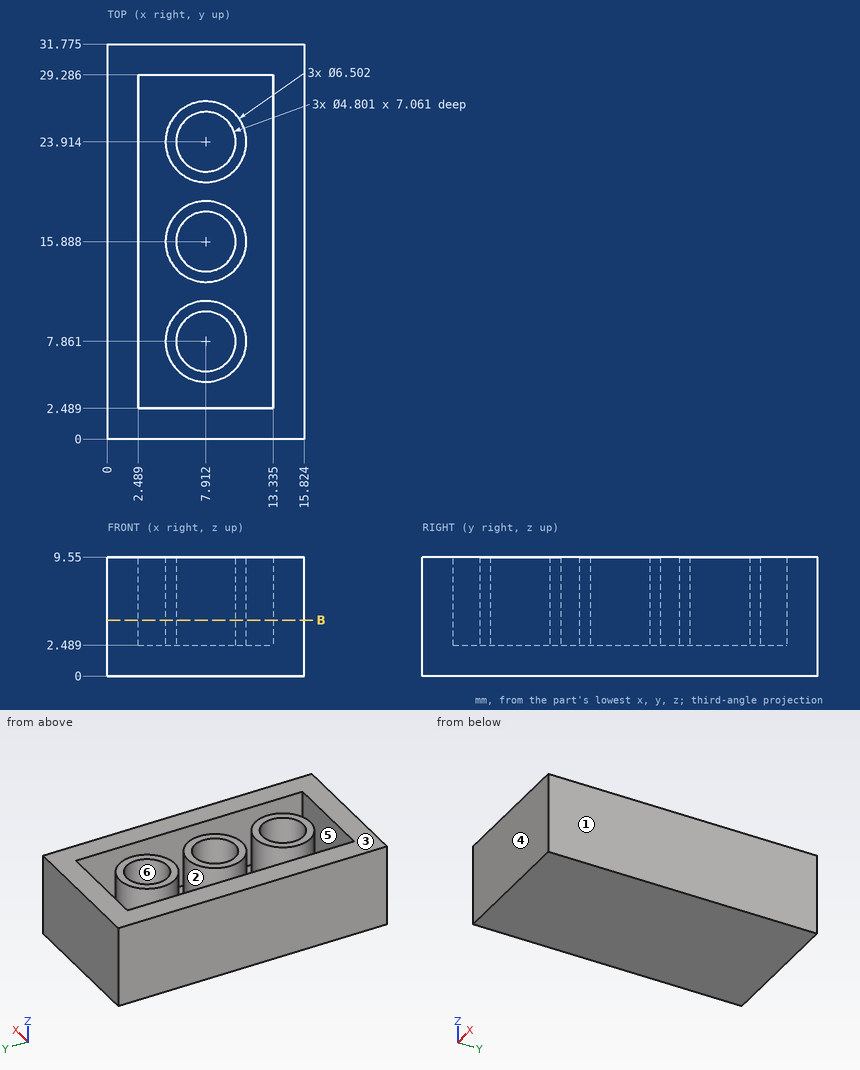
Answer from the drawing. Dimensions are ordinates in mm from the lowest x, y and z of the part. A direction names the side the tool comes from. Round coordinates to 2 decimals unless told otherwise and drop trailing zeros. Order: outer loops, then holes, each group sorted by start corner. A loop starts at its lowest first (then second) coordinate and runs counter-clockwise, first axis right, second up.
1) A flat-ended cylindrical pin translates along its axis: pin 1 (1.4 mm diameter, centred on x = 8.5, y = 25, fed in from +Z). Find the tip coordinate at first contact, or state that the pin passes through.
2) The part is cut by section B-B on z = 4.5. Write down the section's boundary in (x, y) (1 decimal).
3) Straight lines are drawn through the part: L1, parallel to X at y = 8, z = 9 (1 decimal); L2, parallel to Y at x = 11.5, z = 8.75 (1 decimal); L3, parallel to X at y = 12.5, z = 3 (1 decimal). For each, find the intervals that lie inside material, in ascending order.
4) For the marked faces 1 and 2, determine the directions among +Z, -Z, +X, -X, +Y, -Y from which every point of the face is accessible in a straight line to the end or side of a thin tool.
5) The mould has two halves that part along Y. Classify the marked faces 3, 4, 5 and 6: released by +Y, released by -Y, zero draft, split by the parting line, or undercut.
Resolved:
1. pin 1: stops at z = 2.49
2. outline: (0, 0) - (15.8, 0) - (15.8, 31.8) - (0, 31.8) - close; circle Ø6.5 at (7.9, 7.9); circle Ø6.5 at (7.9, 15.9); circle Ø6.5 at (7.9, 23.9); hole (2.5, 2.5) - (13.3, 2.5) - (13.3, 29.3) - (2.5, 29.3) - close; hole circle Ø4.8 at (7.9, 7.9); hole circle Ø4.8 at (7.9, 15.9); hole circle Ø4.8 at (7.9, 23.9)
3. L1: x = 0 to 2.5, 4.7 to 5.5, 10.3 to 11.2, 13.3 to 15.8
3. L2: y = 0 to 2.5, 29.3 to 31.8
3. L3: x = 0 to 2.5, 13.3 to 15.8
4. face 1: +Z, -Z, +X, +Y, -Y
4. face 2: +Z
5. face 3: zero draft
5. face 4: released by -Y
5. face 5: undercut
5. face 6: undercut
